Verification items for the finished model (mm, model axes). Face numbers are marked on the shaded views. Round coordinates to 2 decimals unless told otherwise and drop trailing zeros. Order: outer loops, then holes, each group sorted by start corner. A loop starts at its lowest first (then second) coordinate and runs counter-clockwise, first axis right, second up. Notation, with made-up numbers: M 50,-5 L 62,-5 A18 cw 62,17 Z; hole C 5.25,-6 d5. An arc over 180 degrees is marked long. Use one line per item in the form item = value. Start each with the question number.
Item 1: Thickness scan on probe 1 along Y at (x, z) = (0, 39) (3 decimals); probe 2 along Y at (x, z) = (0, 26) (3 decimals); probe 3 along Z at (x, y) = (7, 1). Record the ranges inside material, lowest first. Write a range as [from, to].
Item 2: Cross-section at D-D on x = -12.5. Enter the section's corners in (y, z).
Item 3: Cross-section at A-A on x = 0. Enter the section's corners in (y, z) (3 decimals).
Item 4: Cross-section at C-C on z = 32. Enter the section's corners in (x, y) (3 decimals), then the cut area to 3 significant figures.
Item 5: Go/stop test with flat-tipped pins: pin 1 Ø4 at (x, y) = (-1, -0.5) entering from +Z; pin 2 Ø10 at (y, z) = (10.5, 69.5) entering from -X; pin 3 Ø12 at (x, y) = (-8.5, -0.5) entering from -Z; pin 4 Ø2.5 at (x, y) = (0, 0) entering from +Z. Record where each tip stops, or that it passes through.
Item 6: Release check for a two-part mould opening along X. For the marked faces 1 and 2 record: +X half, -X half, draft (parallel to the pull), parting line (faces both ways), or undercut.
Autodesk Fusion 360 part; units mm, degrees
sketch "Sketch1" plane through (0, 0, 0) normal (0, 0, 1) x (1, 0, 0)
  circle A0 centre (0, 0) radius 19.305
  circle A1 centre (0, 0) radius 16.25
  dimension "d1" = 38.61
  dimension "d9" = 32.5
extrude "Extrude1" add sketch "Sketch1" along normal blind 80 makes body 1
ref_plane "WorkPlane1" through (0, 0, 40) normal (0, 0, 1) x (1, 0, 0)
sketch "Sketch2" plane through (0, 0, 40) normal (0, 0, 1) x (1, 0, 0)
  circle A0 centre (0, 0) radius 18.6687
  circle A1 centre (0, 0) radius 2.15
  dimension "d6" = 4.3
extrude "Extrude2" add sketch "Sketch2" along normal mid plane 5 separate body makes body 2
combine "Combine1" operation add target body 1 tool bodies 2
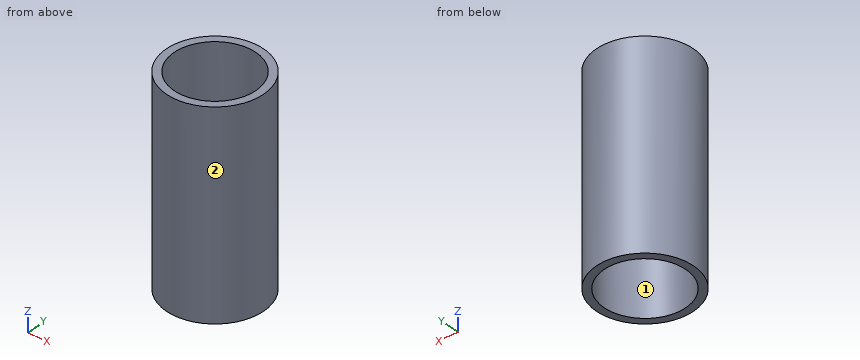
Output values:
q1.probe_1 = [-19.305, -2.15], [2.15, 19.305]
q1.probe_2 = [-19.305, -16.25], [16.25, 19.305]
q1.probe_3 = [37.5, 42.5]
q2.outline = M -14.71,0 L -10.38,0 L -10.38,37.5 L 10.38,37.5 L 10.38,0 L 14.71,0 L 14.71,80 L 10.38,80 L 10.38,42.5 L -10.38,42.5 L -10.38,80 L -14.71,80 Z
q3.outline = M -19.305,0 L -16.25,0 L -16.25,37.5 L -2.15,37.5 L -2.15,42.5 L -16.25,42.5 L -16.25,80 L -19.305,80 Z; M 2.15,37.5 L 16.25,37.5 L 16.25,0 L 19.305,0 L 19.305,80 L 16.25,80 L 16.25,42.5 L 2.15,42.5 Z
q4.outline = C 0,0 d38.61; hole C 0,0 d32.5
q4.area = 341 mm2
q5.pin_1 = 42.5
q5.pin_2 = -18.5
q5.pin_3 = 37.5
q5.pin_4 = through
q6.face_1 = undercut
q6.face_2 = parting line
